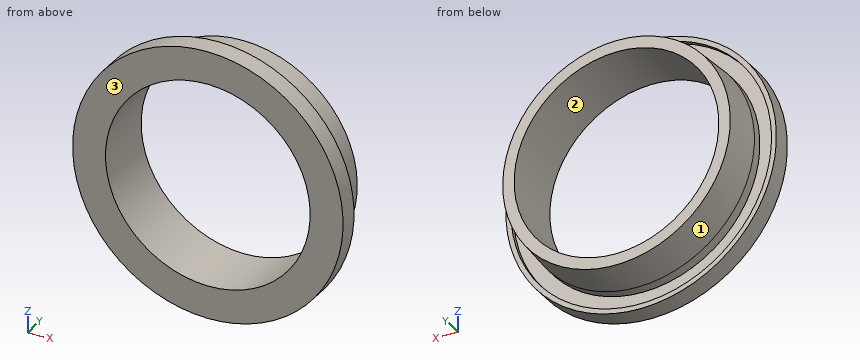
from build123d import *

# Parameters (mm, degrees)
SKETCH1_R               = 69.375
SKETCH1_R_2             = 66.875
BOSS_EXTRUDE1_DEPTH     = 2.5
BOSS_EXTRUDE2_START     = -7.5
SKETCH2_R               = 69.375
BOSS_EXTRUDE2_DEPTH     = 7.5
SKETCH3_R               = 59.5
BOSS_EXTRUDE3_DEPTH     = 25
CHAMFER1_SIZE           = 20
CHAMFER1_SIZE2          = 1.135682303
CUT_EXTRUDE1_DEPTH      = 104.353912601
CUT_EXTRUDE1_DEPTH_BACK = 104.353912601
SKETCH4_R               = 52.5


with BuildPart() as part:
    # Sketch1 → Boss-Extrude1 (new body)
    with BuildSketch(Plane(origin=(0, 0, 0), x_dir=(1, 0, 0), z_dir=(0, 1, 0))):
        with Locations(Location((0, 0, 0), (0, 0, 270))):
            Circle(SKETCH1_R)
        with Locations(Location((0, 0, 0), (0, 0, 270))):
            Circle(SKETCH1_R_2, mode=Mode.SUBTRACT)
    extrude(amount=BOSS_EXTRUDE1_DEPTH)

    # Sketch2 → Boss-Extrude2 (add)
    with BuildSketch(Plane(origin=(0, 0, 0), x_dir=(1, 0, 0), z_dir=(0, 1, 0)).offset(BOSS_EXTRUDE2_START)):
        with Locations(Location((0, 0, 0), (0, 0, 270))):
            Circle(SKETCH2_R)
    extrude(amount=BOSS_EXTRUDE2_DEPTH)

    # Sketch3 → Boss-Extrude3 (add)
    with BuildSketch(Plane(origin=(0, 0, 0), x_dir=(1, 0, 0), z_dir=(0, 1, 0))):
        with Locations(Location((0, 0, 0), (0, 0, 270))):
            Circle(SKETCH3_R)
    extrude(amount=BOSS_EXTRUDE3_DEPTH)

    # Chamfer1
    chamfer1_edges = [part.edges().sort_by_distance(p)[0] for p in [
        (0, 25, -59.5),
    ]]
    chamfer1_side = [part.faces().sort_by_distance(p)[0] for p in [
        (0, 12.5, -59.5),
    ]]
    chamfer(chamfer1_edges, length=CHAMFER1_SIZE, length2=CHAMFER1_SIZE2, reference=chamfer1_side[0])

    # Sketch4 → Cut-Extrude1 (cut, two sides: drawn at the far end of the back side and taken through both)
    with BuildSketch(Plane(origin=(0, 25, 0), x_dir=(1, 0, 0), z_dir=(0, 1, 0)).offset(-CUT_EXTRUDE1_DEPTH_BACK)):
        with Locations(Location((0, 0, 0), (0, 0, 270))):
            Circle(SKETCH4_R)
    extrude(amount=CUT_EXTRUDE1_DEPTH + CUT_EXTRUDE1_DEPTH_BACK, mode=Mode.SUBTRACT)


solid = part.part
Check sheet for the modelled part. Datum: model origin and axes. Units: mm. Face numbers are marked on the shaded views. Give positions to 0.01 mm unless a question says otherwise; leave off trailing zeros. Write each loop counter-clockwise with the first axis right and the second up, starting at its lowest first coordinate (ties: lowest second). Pieces come first, ordered by that corner, then holes. Notation, with made-up numbers: (37.25, -5) -> (45.25, -5) arc R23 ccw to (45.25, 16) -> close; hole circle Ø2 at (-27.5, -34.5). An arc over 180 degrees is marked (long way). Write item = value, one per line.
Item 1: Sectioned sample at A-A on x = 0. Record the boundary of the cut face in (y, z) (3 decimals).
Output:
outline = (-7.5, -69.375) -> (2.5, -69.375) -> (2.5, -66.875) -> (0, -66.875) -> (0, -59.5) -> (5, -59.5) -> (25, -58.364) -> (25, -52.5) -> (-7.5, -52.5) -> close; (-7.5, 52.5) -> (25, 52.5) -> (25, 58.364) -> (5, 59.5) -> (0, 59.5) -> (0, 66.875) -> (2.5, 66.875) -> (2.5, 69.375) -> (-7.5, 69.375) -> close
Item 2: Sectioned sample at D-D on y = 8. Record the boundary of the cut face in (x, z), and give its area (3 significant figures).
Output:
outline = circle Ø118.66 at (0, 0); hole circle Ø105 at (0, 0)
area = 2,400 mm^2
Item 3: Release check for a two-part mould opening along X. For the marked faces 1, 2 and 3 record: +X half, -X half, draft (parallel to the pull), parting line (faces both ways), or undercut.
Output:
face_1 = parting line
face_2 = undercut
face_3 = draft
Item 4: Scan lines: probe 1 along X at (y, z) = (1.65, 0) (3 decimals); probe 2 along Z at (x, y) = (35, -2.5); probe 3 along Z at (x, y) = (-37.5, 16). Record each from-to range of solid material in increasing order. Write a range as from..to.
Output:
probe_1 = -69.375..-66.875, -59.5..-52.5, 52.5..59.5, 66.875..69.375
probe_2 = -59.9..-39.13, 39.13..59.9
probe_3 = -45.39..-36.74, 36.74..45.39
Item 5: Gauge pin test, flat ends, axial feed: pin 1 (5 mm diameter, centred on x = -31, y = 21.5, fed in from +Z); pin 2 (2 mm diameter, centred on x = 4.5, y = 17, fed in from +Z); pin 3 (10 mm diameter, centred on x = 16, y = -2, fed in from +Z); pin 4 (4 mm diameter, centred on x = -46, z = 38, fed in from +Y). Record the tip position at first contact, or that the pin passes through.
Output:
pin_1 = 51.17
pin_2 = 58.74
pin_3 = 68.5
pin_4 = 25
Item 6: Sectioned sample at C-C on y = 23. Record the boundary of the cut face in (x, z).
Output:
outline = circle Ø116.96 at (0, 0); hole circle Ø105 at (0, 0)
Item 7: Sectioned sample at B-B on z = 0. Record the boundary of the cut face in (x, y) (3 decimals), and give its area (3 significant figures).
Output:
outline = (-69.375, -7.5) -> (-52.5, -7.5) -> (-52.5, 25) -> (-58.364, 25) -> (-59.5, 5) -> (-59.5, 0) -> (-66.875, 0) -> (-66.875, 2.5) -> (-69.375, 2.5) -> close; (52.5, -7.5) -> (69.375, -7.5) -> (69.375, 2.5) -> (66.875, 2.5) -> (66.875, 0) -> (59.5, 0) -> (59.5, 5) -> (58.364, 25) -> (52.5, 25) -> close
area = 593 mm^2
